Could you check a few things on this model? Use its own coordinates, in mm. A direction names the side the tool comes from. Coordinates: 2 decimals unless noted, no trailing zeros. Order: outer loops, then holes, each group sorted by start corner. A loop starts at its lowest first (then second) coordinate and runs counter-clockwise, first axis right, second up. Notation, with made-up numbers: (30.25, -0.75) -> (51.25, -0.75) arc R13 ccw to (51.25, 6.25) -> close; hole circle Ø1 at (56, 52.25). An arc over 180 degrees is marked (long way). Use a Markdown table: item, result. Add a question column.
1) Which directions (+Z, -Z, +X, -X, +Y, -Y) give clear straight access to the entire face, cutting with the end or side of a thin tool? Please do faces 1 (the cylindrical face through (-1.887, 3.219, -15.805)), 2 (the cylindrical face through (-4.823, 3.219, -18.338)).
2) Will these pins go through, and if not, where does the flat tip stop? pin 1 Ø1 at (y, z) = (1, -5) entering from +X; pin 2 Ø1.5 at (y, z) = (1, 11) entering from +X; pin 3 Ø1.5 at (x, y) = (-1.5, 2) entering from +Z.
3) If we section it at B-B (x = 13): Write out the boundary of the cut face in (y, z).
4) If we section it at D-D (y = 2.75): Give the number of separate pieces and of enclosed holes in the cut face, plus the area to 3 significant figures.
5) If we section it at A-A (z = -8.25): Write out the boundary of the cut face in (x, y), plus the area to 3 significant figures.
6) If I drill on L1, parallel to X at y = 1.75, z = -8.25; L2, parallel to X at y = 1.25, z = -9.5; L3, parallel to Z at x = 7, y = 4.5, over which ranges is the centre line in solid material (lowest first)? Write a range as [from, to].
7) If we section it at C-C (z = 6): Write out the boundary of the cut face in (x, y), plus the area to 3 significant figures.
8) Thinking about a two-plate mould opening in X: for faces 3 (the flat face through (5.119, 3.219, -12.634)), 4 (the cylindrical face through (0.526, 3.131, 18.169)), 5 (the flat face through (10.2, 3.1, 5.9)), 6 (the cylindrical face through (-14.213, 3.131, -13.714)), which applies, +X half, -X half, draft (parallel to the pull), parting line (faces both ways), or undercut?
```python
from build123d import *

# Parameters (mm, degrees)
SKETCH1_R           = 7.75
SKETCH1_R_2         = 1.75
BOSS_EXTRUDE1_DEPTH = 6.35
CUT_EXTRUDE1_DEPTH  = 7.35


with BuildPart() as part:
    # Sketch1 → Boss-Extrude1 (new body)
    with BuildSketch(Plane(origin=(0, 0, 0), x_dir=(1, 0, 0), z_dir=(0, 1, 0))):
        with BuildLine():
            Line((-17.135648679, 6.681090334), (-3.5, -18.055952583))
            ThreePointArc((-3.5, -18.055952583), (-2.361702731, -19.252086758), (-0.782543458, -19.734490765))
            ThreePointArc((-0.782543458, -19.734490765), (0, -19.75), (0.782543458, -19.734490765))
            ThreePointArc((0.782543458, -19.734490765), (2.361702731, -19.252086758), (3.5, -18.055952583))
            Line((3.5, -18.055952583), (17.135648679, 6.681090334))
            ThreePointArc((17.135648679, 6.681090334), (17.539259633, 8.282201146), (17.104001725, 9.875))
            ThreePointArc((17.104001725, 9.875), (0, 19.75), (-17.104001725, 9.875))
            ThreePointArc((-17.104001725, 9.875), (-17.539259633, 8.282201146), (-17.135648679, 6.681090334))
        make_face()
        with Locations(Location((0, 0, 0), (0, 0, 270))):  # turned: the seam where the file's is
            Circle(SKETCH1_R, mode=Mode.SUBTRACT)
        with Locations(Location((-14.289419162, 8.25, 0), (0, 0, 270))):  # turned: the seam where the file's is
            Circle(SKETCH1_R_2, mode=Mode.SUBTRACT)
        with Locations(Location((0, -16.5, 0), (0, 0, 270))):  # turned: the seam where the file's is
            Circle(SKETCH1_R_2, mode=Mode.SUBTRACT)
        with Locations(Location((14.289419162, 8.25, 0), (0, 0, 270))):  # turned: the seam where the file's is
            Circle(SKETCH1_R_2, mode=Mode.SUBTRACT)
    extrude(amount=BOSS_EXTRUDE1_DEPTH)

    # Sketch2 → Cut-Extrude1 (cut, through all)
    with BuildSketch(Plane(origin=(0, 6.35, 0), x_dir=(1, 0, 0), z_dir=(0, 1, 0))):
        with BuildLine():
            Line((3.147914252, 13.43813294), (7.146291664, 11.807764247))
            ThreePointArc((7.146291664, 11.807764247), (9.680193531, 12.584478285), (9.426519569, 15.222582318))
            ThreePointArc((9.426519569, 15.222582318), (9.362829603, 16.466865659), (10.592172309, 16.669384685))
            ThreePointArc((10.592172309, 16.669384685), (7.457105532, 18.288085659), (4.084045388, 19.323122762))
            ThreePointArc((4.084045388, 19.323122762), (4.821258852, 18.318725553), (3.905659686, 17.473754778))
            ThreePointArc((3.905659686, 17.473754778), (1.879612558, 15.765224297), (3.147914252, 13.43813294))
        make_face()
    cut_extrude1 = extrude(amount=-CUT_EXTRUDE1_DEPTH, mode=Mode.SUBTRACT)

    # Mirror1: Cut-Extrude1 across plane
    add(cut_extrude1.mirror(Plane(origin=(0, 0, 0), x_dir=(0, 0, 1), z_dir=(1, 0, 0))), mode=Mode.SUBTRACT)


solid = part.part
```
Answer sheet:
| question | item | result |
|---|---|---|
| 1 | face 1 | +Y, -Y |
| 1 | face 2 | -X, +Y, -Y |
| 2 | pin 1 | x = 16.48 |
| 2 | pin 2 | x = 7.8 |
| 2 | pin 3 | z = 19.74 |
| 3 | outline | (0, -14.87) -> (6.35, -14.87) -> (6.35, -9.43) -> (0, -9.43) -> close; (0, -7.07) -> (6.35, -7.07) -> (6.35, 0.82) -> (0, 0.82) -> close |
| 4 | separate pieces | 1 |
| 4 | enclosed holes | 4 |
| 4 | area | 569 mm2 |
| 5 | outline | (-17.54, 0) -> (-16.04, 0) -> (-16.04, 6.35) -> (-17.54, 6.35) -> close; (-12.54, 0) -> (12.54, 0) -> (12.54, 6.35) -> (-12.54, 6.35) -> close; (16.04, 0) -> (17.54, 0) -> (17.54, 6.35) -> (16.04, 6.35) -> close |
| 5 | area | 178 mm2 |
| 6 | L1 | [-17.54, -16.04], [-12.54, 12.54], [16.04, 17.54] |
| 6 | L2 | [-17.29, -15.51], [-13.06, 13.06], [15.51, 17.29] |
| 6 | L3 | [-11.87, -3.33], [3.33, 11.71] |
| 7 | outline | (-10.15, 0) -> (-4.91, 0) -> (-4.91, 6.35) -> (-10.15, 6.35) -> close; (4.91, 0) -> (10.15, 0) -> (10.15, 6.35) -> (4.91, 6.35) -> close |
| 7 | area | 66.6 mm2 |
| 8 | face 3 | undercut |
| 8 | face 4 | undercut |
| 8 | face 5 | +X half |
| 8 | face 6 | -X half |
